Part model, mm, in its own coordinate system. Face numbers are marked on the shaded views. A direction names the side the tool comes from. Coordinates: 2 decimals unless noted, no trailing zeros. Order: outer loops, then holes, each group sorted by start corner. A loop starts at its lowest first (then second) coordinate and runs counter-clockwise, first axis right, second up.
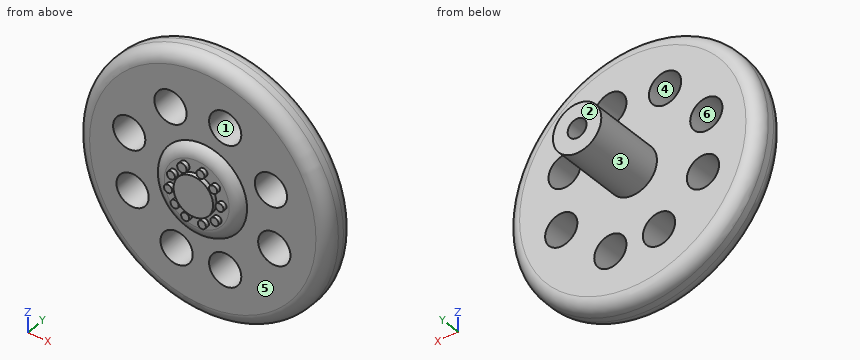
```python
from build123d import *

# Parameters (mm, degrees)
F0_R      = 15.625
F1_DEPTH  = 4
F2_R      = 2.4511
F3_DEPTH  = 1.55
F4_R      = 3
F5_DEPTH  = 9.1
F6_R      = 1.171580863
F7_DEPTH  = 6
F8_R      = 5.5
F9_DEPTH  = 1
F11_R     = 0.5
F11_R_2   = 0.5786516817
F12_DEPTH = 0.5
F13_R     = 2
F14_DEPTH = 25.4


# Not quite as in the source:
# - a fillet or chamfer that OpenCascade refuses, or shapes differently, is made with other operations: its cross-section is extruded or revolved along the edge and cut away or added


with BuildPart() as f1:
    # F0 (on Front) → F1 (new body)
    with BuildSketch(Plane.XZ):
        Circle(F0_R)
    extrude(amount=F1_DEPTH)

    # F2 (on face) → F3 (join)
    with BuildSketch(Plane.XZ.offset(4)):
        Circle(F2_R)
    extrude(amount=F3_DEPTH)

    # F4 (on face) → F5 (join)
    with BuildSketch(Plane(origin=(0, 0, 0), x_dir=(-1, 0, 0), z_dir=(0, 1, 0))):
        Circle(F4_R)
    extrude(amount=F5_DEPTH)

    # F6 (on face) → F7 (cut)
    with BuildSketch(Plane(origin=(0, 9.1, 0), x_dir=(-1, 0, 0), z_dir=(0, 1, 0))):
        Circle(F6_R)
    extrude(amount=-F7_DEPTH, mode=Mode.SUBTRACT)

    # F8 (on face) → F9 (join)
    with BuildSketch(Plane.XZ.offset(4)):
        Circle(F8_R)
    extrude(amount=F9_DEPTH)

    # F10: fillet of radius 1.58242 on 3 edges, made by hand

    # F10_s1 → F10_t2 (revolve, cut)
    with BuildSketch(Plane.XY):
        with BuildLine():
            ThreePointArc((15.625, -2.41758), (15.1615199127, -3.5365199127), (14.04258, -4))
            Line((14.04258, -4), (15.625, -4))
            Line((15.625, -4), (15.625, -2.41758))
        make_face()
    revolve(axis=Axis((0, -4, 0), (0, -1, 0)), mode=Mode.SUBTRACT)

    # F10_s3 → F10_t4 (revolve, cut)
    with BuildSketch(Plane.XY):
        with BuildLine():
            ThreePointArc((15.625, -1.58242), (15.1615199127, -0.4634800873), (14.04258, 0))
            Line((14.04258, 0), (15.625, 0))
            Line((15.625, 0), (15.625, -1.58242))
        make_face()
    revolve(axis=Axis((0, 0, 0), (0, -1, 0)), mode=Mode.SUBTRACT)

    # F10_s5 → F10_t6 (revolve, cut)
    with BuildSketch(Plane.XY):
        with BuildLine():
            ThreePointArc((5.5, -4), (4.9181603337, -4.7263363014), (4.0286604743, -5))
            Line((4.0286604743, -5), (5.5, -5))
            Line((5.5, -5), (5.5, -4))
        make_face()
    revolve(axis=Axis((0, -5, 0), (0, -1, 0)), mode=Mode.SUBTRACT)

    # F11 (on face) → F12 (join)
    with BuildSketch(Plane.XZ.offset(5)):
        with Locations((-2.8265540022, 1.3354053954)):
            Circle(F11_R)
        with Locations((-1.4595896937, 2.8208354488)):
            Circle(F11_R_2)
        with Locations((2.4141243193, 1.8303584075)):
            Circle(F11_R)
        with Locations((3.2077198848, 0)):
            Circle(F11_R)
        with Locations((2.5885446352, -1.9824508684)):
            Circle(F11_R)
        with Locations((1.0188785489, -3.0214018971)):
            Circle(F11_R)
        with Locations((-1.0465403436, -2.928553993)):
            Circle(F11_R)
        with Locations((-3.1790773666, -0.4500864609)):
            Circle(F11_R)
        with Locations((0.8419207879, 2.9949534219)):
            Circle(F11_R)
        with Locations((-2.3607159965, -1.9545760006)):
            Circle(F11_R)
    extrude(amount=F12_DEPTH)

    # F13 (on face) → F14 (cut)
    with BuildSketch(Plane.XZ.offset(4)):
        with Locations((-4.0041380562, 8.2640713081)):
            Circle(F13_R)
        with Locations((2.7820917312, 8.610307239)):
            Circle(F13_R)
        with Locations((-9.1284336522, 2.9320335016)):
            Circle(F13_R)
        with Locations((8.4603661671, 3.555258736)):
            Circle(F13_R)
        with Locations((8.8758496568, -3.3694657031)):
            Circle(F13_R)
        with Locations((2.7820917312, -8.5630090907)):
            Circle(F13_R)
        with Locations((-3.2498515921, -8.4628218188)):
            Circle(F13_R)
        with Locations((-8.7129501626, -3.8541962858)):
            Circle(F13_R)
    extrude(amount=-F14_DEPTH, mode=Mode.SUBTRACT)


solid = f1.part
```
(1) Slice it at B-B, the plane x = -8.5. State how many separate pieces and enclosed holes the cut face has, then the cut area to 3 significant figures.
(2) Drop flat-ended pins along their axis: pin 1 (4.5 mm diameter, centred on x = 8.88, z = -3.37, fed in from -Y); pin 2 (2 mm diameter, centred on x = 9, z = 10.5, fed in from +Y); pin 3 (2.5 mm diameter, centred on x = -0.5, z = 0, fed in from +Y); pin 4 (0.8 mm diameter, centred on x = 1, z = -3, fed in from -Y). Give the stop position or say it passes through.
(3) Probe line 1 (X direction, y = -2.25, z = -5); line 2 (Z direction, x = 0, y = 5); line 3 (Y direction, x = 8, z = -11). List the from-to ranges inside material, lowest first.
(4) Slice it at D-D, the plane y = -4.5. Give the cut face in (x, z).
(5) Slice it at A-A, the plane y = 4.25. Give the cut face in (x, z).
(6) Tool access for the marked faces 5 and 6: list every direction of +Z, -Z, +X, -X, +Y, -Y with a clear straight run to the whole face (end or side of a thin tool).
(7) Pull direction X, two halves, no side cores. Call the marked faces 1, 2, 3 and 4: +X half, -X half, draft (parallel to the pull), parting line (faces both ways), or undercut.
Here are the results:
1. separate pieces: 3
1. enclosed holes: 0
1. area: 71.2 mm2
2. pin 1: stops at y = -4
2. pin 2: stops at y = 0
2. pin 3: stops at y = 9.1
2. pin 4: stops at y = -5.5
3. line 1: x = -14.8 to -10.35, -7.07 to 7.72, 10.03 to 14.8
3. line 2: z = -3 to -1.17, 1.17 to 3
3. line 3: y = -4 to 0
4. outline: circle Ø10.37 at (0, 0)
5. outline: circle Ø6 at (0, 0); hole circle Ø2.34 at (0, 0)
6. face 5: -Y
6. face 6: +Y, -Y
7. face 1: undercut
7. face 2: draft
7. face 3: parting line
7. face 4: undercut
